from build123d import *

# Parameters (mm, degrees)
BOSS_EXTRUDE1_DEPTH = 63.5
SKETCH2_R           = 14.2875
CUT_EXTRUDE1_DEPTH  = 51.8


with BuildPart() as part:
    # Sketch1 → Boss-Extrude1 (new body)
    with BuildSketch(Plane.XY):
        Polygon((0, 0), (0, 101.6), (3.175, 101.6), (3.175, 3.175), (50.8, 3.175), (50.8, 0), align=None)
    extrude(amount=BOSS_EXTRUDE1_DEPTH)

    # Sketch2 → Cut-Extrude1 (cut, through all)
    with BuildSketch(Plane.ZY):
        with Locations((31.75, 63.5)):
            Circle(SKETCH2_R)
    extrude(amount=-CUT_EXTRUDE1_DEPTH, mode=Mode.SUBTRACT)


solid = part.part
The listing builds one solid part. Answer for the finished solid, in the listing's coordinates (mm). A direction names the side the tool comes from. Give positions to 0.01 mm unless a question says otherwise; leave off trailing zeros. Write each loop counter-clockwise with the first axis right and the second up, starting at its lowest first coordinate (ties: lowest second). Pieces come first, ordered by that corner, then holes.
1) Given P1, Ø1, axis at x = 12, z = 33.5, coming from the -Y side; P2, Ø1, axis at x = 45, z = 50.5, coming from the +Y side (3 decimals), each flat-ended and moving along its own axis, determine where each tip first touches the part or whether it passes through.
2) For a pull along Y with two mould halves and no side action, classify faces 1 (the face through (50.8, 2, 31)), 2 (the face through (27, 3.175, 31)), 3 (the face through (1.565, 77.666, 29.89)) as pulls with the +Y half, pulls with the -Y half, needs draft (parallel to the pull), parting line crosses it, or undercut.
3) Find the intervals of material crossed by L1, parallel to Z at x = 1, y = 63; L2, parallel to Y at x = 1.8, z = 31.75; L3, parallel to Y at x = 44.5, z = 26 (3 decimals), in increasing order.
4) A tool of negligible diameter and unlimited length cuts with its end or side. For faces 4 (the face through (26, 0, 31)), 5 (the face through (3.175, 42, 31)), from which of +Z, -Z, +X, -X, +Y, -Y can it reach the whole face along a straight path? Write none if from no direction.
5) Section B-B (z = 31.75) is taken. Write down the section's boundary in (x, y) (1 decimal).
6) Section D-D (y = 86.5) is taken. Write down the section's boundary in (x, z) (3 decimals).
7) Section C-C (z = 9) is taken. Write down the section's boundary in (x, y) (3 decimals).
8) Section A-A (y = 63.5) is taken. Write down the section's boundary in (x, z) (1 decimal).
Response:
1. P1: stops at y = 0
1. P2: stops at y = 3.175
2. face 1: needs draft
2. face 2: pulls with the +Y half
2. face 3: undercut
3. L1: z = 0 to 17.47, 46.03 to 63.5
3. L2: y = 0 to 49.21, 77.79 to 101.6
3. L3: y = 0 to 3.175
4. face 4: +Z, -Z, +X, -X, -Y
4. face 5: +Z, -Z, +X, +Y
5. outline: (0, 0) - (50.8, 0) - (50.8, 3.2) - (3.2, 3.2) - (3.2, 49.2) - (0, 49.2) - close; (0, 77.8) - (3.2, 77.8) - (3.2, 101.6) - (0, 101.6) - close
6. outline: (0, 0) - (3.175, 0) - (3.175, 63.5) - (0, 63.5) - close
7. outline: (0, 0) - (50.8, 0) - (50.8, 3.175) - (3.175, 3.175) - (3.175, 101.6) - (0, 101.6) - close
8. outline: (0, 0) - (3.2, 0) - (3.2, 17.5) - (0, 17.5) - close; (0, 46) - (3.2, 46) - (3.2, 63.5) - (0, 63.5) - close
